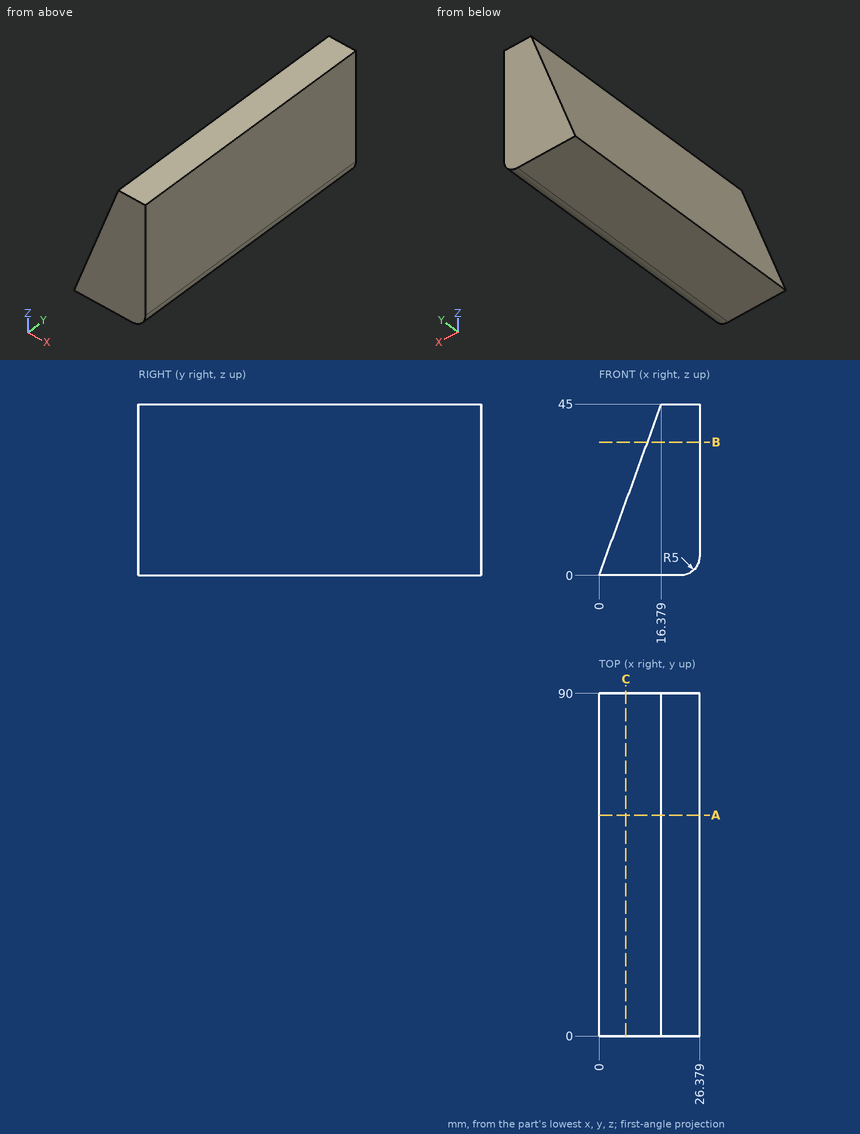
Drawing for the job (mm, zero at the part's lowest x, y, z). Give positions to 0.01 mm unless a question says otherwise; leave off trailing zeros. Loops run counter-clockwise (first coordinate to the right, second up) from the corner with the lowest first, then second, coordinate; pieces in that order, holes last. Notation, with made-up numbers: M 81.25,27 L 86.25,27 A20 cw 86.25,50 Z; hole C -27.75,13 d9. An arc over 180 degrees is marked long. One line per question, with ' | ' between items. Start each with the question number.
1. Saw through at A-A on y = 58. Give the cut face in (x, z), plus the area to 3 significant figures.
2. Saw through at B-B on z = 35. Give the cut face in (x, y), plus the area to 3 significant figures.
3. Probe L1, parallel to X at y = 11, z = 11; L2, parallel to X at y = 70, z = 13.5; L3, parallel to Z at x = 23.25, y = 67. List the from-to ranges inside material, lowest first. Write a range as from..to.
4. Flat gauge pins, fed straight in: pin 1 (10 mm diameter, centred on x = 6, z = 14.5, fed in from -Y); pin 2 (8 mm diameter, centred on y = 81, z = 19.5, fed in from -X); pin 3 (5 mm diameter, centred on y = 44.5, z = 10.5, fed in from -X). Where does each tip first touch, or does it go through?
5. Saw through at C-C on x = 7. Give the cut face in (y, z).
Result sheet:
1) outline: M 0,0 L 21.38,0 A5 ccw 26.38,5 L 26.38,45 L 16.38,45 Z | area: 813 mm^2
2) outline: M 12.74,0 L 26.38,0 L 26.38,90 L 12.74,90 Z | area: 1,230 mm^2
3) L1: x = 4..26.38 | L2: x = 4.91..26.38 | L3: z = 0.36..45
4) pin 1: stops at y = 0 | pin 2: stops at x = 5.64 | pin 3: stops at x = 2.91
5) outline: M 0,0 L 90,0 L 90,19.23 L 0,19.23 Z
